```python
from build123d import *

# Parameters (mm, degrees)
SKETCH1_W            = 230
SKETCH1_H            = 122
BOSS_EXTRUDE1_DEPTH  = 5
SKETCH2_W            = 20
SKETCH2_H            = 10
BOSS_EXTRUDE2_DEPTH  = 5
FILLET1_R            = 2
FILLET1_OF_MIRROR1_R = 2


with BuildPart() as part:
    # Sketch1 → Boss-Extrude1 (new body)
    with BuildSketch(Plane.XY):
        with Locations((115, 61)):
            Rectangle(SKETCH1_W, SKETCH1_H)
    extrude(amount=BOSS_EXTRUDE1_DEPTH)

    # Sketch2 → Boss-Extrude2 (add)
    with BuildSketch(Plane.XY.offset(5)):
        with Locations((30, 127)):
            Rectangle(SKETCH2_W, SKETCH2_H)
        with Locations((70, 127)):
            Rectangle(SKETCH2_W, SKETCH2_H)
        with Locations((110, 127)):
            Rectangle(SKETCH2_W, SKETCH2_H)
        with Locations((150, 127)):
            Rectangle(SKETCH2_W, SKETCH2_H)
        with Locations((190, 127)):
            Rectangle(SKETCH2_W, SKETCH2_H)
    boss_extrude2 = extrude(amount=-BOSS_EXTRUDE2_DEPTH)

    # Fillet1
    fillet1_edges = [part.edges().sort_by_distance(p)[0] for p in [
        (40, 132, 2.5),
        (20, 132, 2.5),
        (80, 132, 2.5),
        (60, 132, 2.5),
        (120, 132, 2.5),
        (100, 132, 2.5),
        (160, 132, 2.5),
        (140, 132, 2.5),
        (200, 132, 2.5),
        (180, 132, 2.5),
    ]]
    fillet(fillet1_edges, radius=FILLET1_R)

    # Mirror1: Boss-Extrude2 across plane
    add(boss_extrude2.mirror(Plane.ZX.offset(61)))

    # Fillet1 of Mirror1
    fillet1_of_mirror1_edges = [part.edges().sort_by_distance(p)[0] for p in [
        (40, -10, 2.5),
        (20, -10, 2.5),
        (80, -10, 2.5),
        (60, -10, 2.5),
        (120, -10, 2.5),
        (100, -10, 2.5),
        (160, -10, 2.5),
        (140, -10, 2.5),
        (200, -10, 2.5),
        (180, -10, 2.5),
    ]]
    fillet(fillet1_of_mirror1_edges, radius=FILLET1_OF_MIRROR1_R)


solid = part.part
```
Source: CAD feature listing. Evaluate the final solid. Frame: model axes, mm. A direction names the side the tool comes from. Round coordinates to 2 decimals unless told otherwise and drop trailing zeros. Loops run counter-clockwise (first coordinate to the right, second up) from the corner with the lowest first, then second, coordinate; pieces in that order, holes last. Notation, with made-up numbers: M 40.25,15.25 L 56.25,15.25 A27 ccw 56.25,49.25 Z; hole C 6.25,76 d11. An arc over 180 degrees is marked long. Put each result on its own line as item: value.
(1) Access query for faces 5 (the face through (40, -4, 3)), 6 (the face through (130, 122, 2)), 7 (the face through (10, 0, 2)). Directions: +Z, -Z, +X, -X, +Y, -Y. A direction counts if a zero-diameter tool reaches every point of the face in a straight line with its end or side. Return the directions, or none.
Solutions:
face 5: +Z, -Z, -Y
face 6: +Z, -Z, +Y
face 7: +Z, -Z, -X, -Y
(2) First-contact query: pin 1 (1.5 mm diameter, centred on y = 127, z = 3.5, fed in from +X); pin 2 (1.5 mm diameter, centred on x = 9.5, z = 2, fed in from -Y); pin 3 (1.5 mm diameter, centred on y = -2.5, z = 3.5, fed in from -X). Flat tips, straight axial feed; report the tip coordinate or a pass-through.
Solutions:
pin 1: x = 200
pin 2: y = 0
pin 3: x = 20
(3) Section A-A, the plane x = 57. Return loops of the section in (y, z), and give its area (3 significant figures).
Solutions:
outline: M 0,0 L 122,0 L 122,5 L 0,5 Z
area: 610 mm²
(4) Ray query, line 1 (X direction, y = 123, z = 0.7); line 2 (Y direction, x = 52, z = 2.25); line 3 (Y direction, x = 20.5, z = 4.5). Return the intervals inside material, ascending. Write a range as [from, to].
Solutions:
line 1: [20, 40], [60, 80], [100, 120], [140, 160], [180, 200]
line 2: [0, 122]
line 3: [-9.32, 131.32]
(5) Pull-direction query (X, two-part tool) for faces 1 (the face through (160, -4, 3)), 2 (the face through (70, -10, 3)), 3 (the face through (200, 126, 3)), 4 (the face through (100, -4, 3)); classes: released by +X, released by -X, zero draft, split by the parting line, or undercut.
Solutions:
face 1: undercut
face 2: zero draft
face 3: released by +X
face 4: undercut
